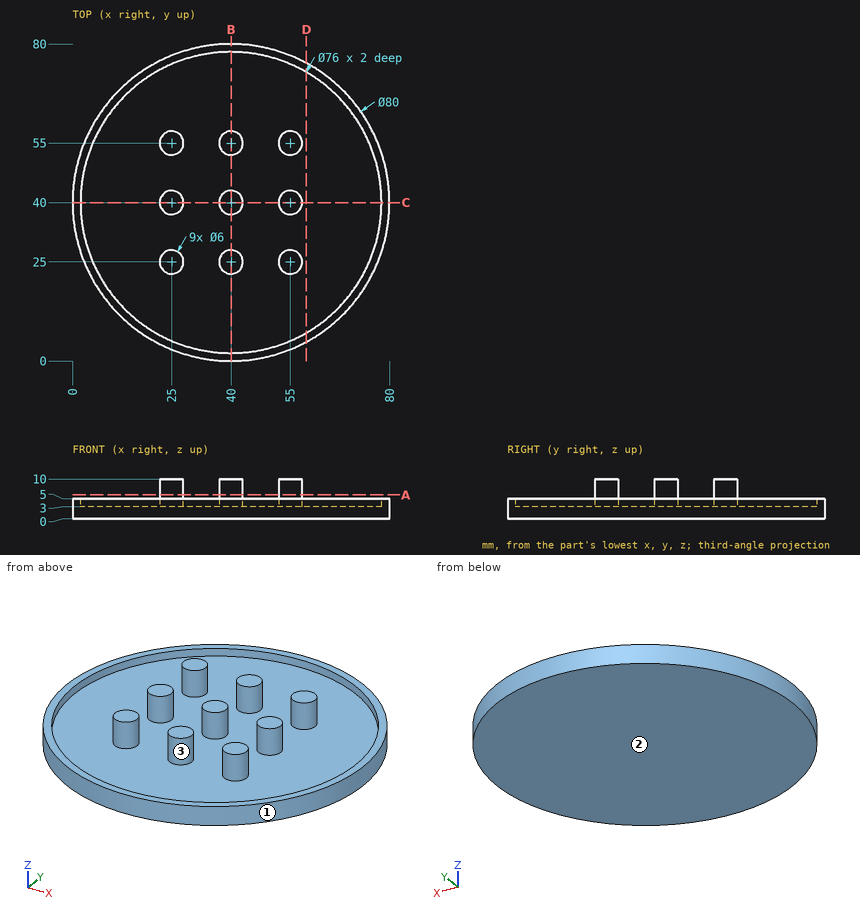
For this review, use the dimensioned drawing (mm, ordinates from the lowest corner) and the shaded views. Round coordinates to 2 decimals unless told otherwise and drop trailing zeros. Loops run counter-clockwise (first coordinate to the right, second up) from the corner with the lowest first, then second, coordinate; pieces in that order, holes last. Notation, with made-up numbers: M -36.5,35.5 L 19.5,35.5 A26 ccw 19.5,59.5 Z; hole C 86.25,23.25 d1. An arc over 180 degrees is marked long. Answer as CSV lines item,"result".
1. Insertion check: pin 1 Ø6 at (y, z) = (72, 4.5) entering from -X; pin 2 Ø12 at (x, y) = (17, 47) entering from +Z; pin 3 Ø1 at (x, z) = (68, 1.5) entering from +Y; pin 4 Ø1 at (x, y) = (62, 66) entering from -Z. Each pin has a flat end and moves straight along its axis. Give the tip position at first contact, or say it passes through.
Outcome:
pin 1,"stops at x = 12.45"
pin 2,"stops at z = 3"
pin 3,"stops at y = 69.05"
pin 4,"stops at z = 0"
2. To check wall thickness, follow L1, parallel to Y at x = 40, z = 4.25; L2, parallel to X at y = 53, z = 8.25; L3, parallel to Y at x = 41, z = 3.75. State the ranges of each line that lie inside material, in increasing order. Write a range as [from, to].
Outcome:
L1,"y = [0, 2], [22, 28], [37, 43], [52, 58], [78, 80]"
L2,"x = [22.76, 27.24], [37.76, 42.24], [52.76, 57.24]"
L3,"y = [0.01, 2.01], [22.17, 27.83], [37.17, 42.83], [52.17, 57.83], [77.99, 79.99]"
3. We need section A-A (z = 6). Count the separate pieces of the cut face and the enclosed holes in it, plus the area to 3 significant figures.
Outcome:
separate pieces,"9"
enclosed holes,"0"
area,"254 mm2"
4. We need section B-B (x = 40). Give the boundary of the cut face in (y, z), plus the area to 3 significant figures.
Outcome:
outline,"M 0,0 L 80,0 L 80,5 L 78,5 L 78,3 L 58,3 L 58,10 L 52,10 L 52,3 L 43,3 L 43,10 L 37,10 L 37,3 L 28,3 L 28,10 L 22,10 L 22,3 L 2,3 L 2,5 L 0,5 Z"
area,"374 mm2"
5. We need section D-D (x = 59). Give the boundary of the cut face in (y, z), plus the area to 3 significant figures.
Outcome:
outline,"M 4.8,0 L 75.2,0 L 75.2,5 L 72.91,5 L 72.91,3 L 7.09,3 L 7.09,5 L 4.8,5 Z"
area,"220 mm2"
6. Draft analysis for pull direction Y (two halves, no side actions). For the marked faces 1, 2 and 3, state which applies: pulls with the +Y half, pulls with the -Y half, needs draft (parallel to the pull), parting line crosses it, or undercut.
Outcome:
face 1,"parting line crosses it"
face 2,"needs draft"
face 3,"undercut"
